from build123d import *

# Parameters (mm, degrees)
SKETCH_1_W          = 50
SKETCH_1_H          = 65
BOSS_EXTRUDE1_DEPTH = 20
SKETCH11_R          = 1.2
CUT_EXTRUDE1_DEPTH  = 28
SKETCH12_R          = 7
CUT_EXTRUDE2_DEPTH  = 15


with BuildPart() as part:
    # 草圖1 → Boss-Extrude1 (new body)
    with BuildSketch(Plane.XY):
        with Locations((2.083333333, 32.5)):
            Rectangle(SKETCH_1_W, SKETCH_1_H)
    extrude(amount=BOSS_EXTRUDE1_DEPTH)

    # Sketch11 → Cut-Extrude1 (cut)
    with BuildSketch(Plane.XY):
        with Locations((-2.916666667, 60.81)):
            Circle(SKETCH11_R)
        with Locations((-2.616666667, 13.19)):
            Circle(SKETCH11_R)
        with Locations((6.783333333, 13.19)):
            Circle(SKETCH11_R)
        with Locations((7.083333333, 60.81)):
            Circle(SKETCH11_R)
        Polygon((4.942250508, 65), (-0.775583841, 65), (-0.775583841, 58), (-8.416666667, 58), (-8.416666667, 16), (12.583333333, 16), (12.583333333, 58), (4.942250508, 58), align=None)
    extrude(amount=CUT_EXTRUDE1_DEPTH, mode=Mode.SUBTRACT)

    # Sketch12 → Cut-Extrude2 (cut)
    with BuildSketch(Plane(origin=(0, 0, 0), x_dir=(1, 0, 0), z_dir=(0, 1, 0))):
        with Locations((-15.232669486, -9.9188946)):
            Circle(SKETCH12_R)
        with Locations((18.767330514, -9.9188946)):
            Circle(SKETCH12_R)
    extrude(amount=CUT_EXTRUDE2_DEPTH, mode=Mode.SUBTRACT)


solid = part.part
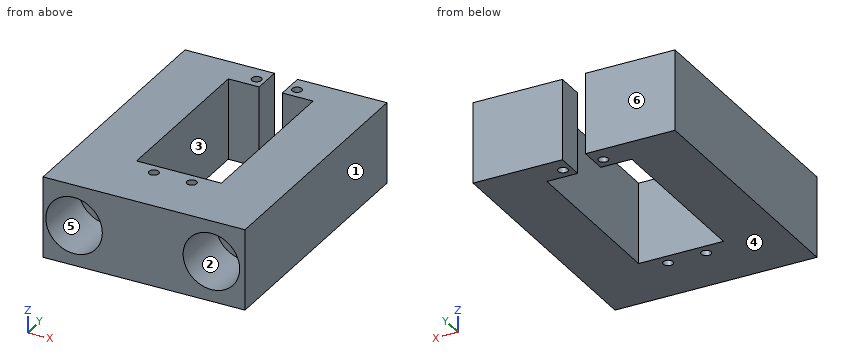
Work out the finished part from the listing and answer in its coordinate system (mm). Face numbers are marked on the shaded views. A direction names the side the tool comes from. Round coordinates to 2 decimals unless told otherwise and drop trailing zeros. Order: outer loops, then holes, each group sorted by start corner. A loop starts at its lowest first (then second) coordinate and runs counter-clockwise, first axis right, second up. Notation, with made-up numbers: M -23.75,63 L 1.25,63 A30 ccw 1.25,101 Z; hole C 22.5,43.5 d10. An arc over 180 degrees is marked long. One line per item, written item: value.
Q1. Determine the mould class of the marked faces 4, 5 and 6 for opening direction Z: released by +Z, released by -Z, zero draft, split by the parting line, or undercut.
Derived:
face 4: released by -Z
face 5: undercut
face 6: zero draft
Q2. Find section D-D on y = 13.19. Write down the section's boundary in (x, z), then the cut area to 3 significant figures.
Derived:
outline: M -22.92,0 L -3.82,0 L -3.82,20 L -22.92,20 Z; M -1.42,0 L 5.58,0 L 5.58,20 L -1.42,20 Z; M 7.98,0 L 27.08,0 L 27.08,20 L 7.98,20 Z; hole C -15.23,9.92 d14; hole C 18.77,9.92 d14
area: 596 mm²
Q3. Straight lines are drawn through the part: line 1 (X direction, y = 57.5, z = 2.25); line 2 (X direction, y = 11, z = 9.5); line 3 (Y direction, x = 6.5, z = 4). For each, find the intervals that lie inside material, in ascending order.
Derived:
line 1: -22.92 to -8.42, 12.58 to 27.08
line 2: -22.92 to -22.22, -8.25 to 11.78, 25.75 to 27.08
line 3: 0 to 12.02, 14.36 to 16, 58 to 59.76, 61.86 to 65
Q4. For the marked faces 1, 2 and 3, determine the directions among +Z, -Z, +X, -X, +Y, -Y from which every point of the face is accessible in a straight line to the end or side of a thin tool.
Derived:
face 1: +Z, -Z, +X, +Y, -Y
face 2: -Y
face 3: +Z, -Z
Q5. A flat-ended cylindrical pin translates along its axis: pin 1 (11 mm diameter, centred on x = 19, z = 9.5, fed in from -Y). Find the tip coordinate at first contact, or state that the pin passes through.
Derived:
pin 1: y = 15
Q6. Find section A-A on y = 23. Write down the section's boundary in (x, z).
Derived:
outline: M -22.92,0 L -8.42,0 L -8.42,20 L -22.92,20 Z; M 12.58,0 L 27.08,0 L 27.08,20 L 12.58,20 Z
Q7. Find section B-B on x = 10.5. Write down the section's boundary in (y, z).
Derived:
outline: M 0,0 L 16,0 L 16,20 L 0,20 Z; M 58,0 L 65,0 L 65,20 L 58,20 Z
Q8. Find section C-C on y = 60.81. Write down the section's boundary in (x, z), then the cut area to 3 significant figures.
Derived:
outline: M -22.92,0 L -4.12,0 L -4.12,20 L -22.92,20 Z; M -1.72,0 L -0.78,0 L -0.78,20 L -1.72,20 Z; M 4.94,0 L 5.88,0 L 5.88,20 L 4.94,20 Z; M 8.28,0 L 27.08,0 L 27.08,20 L 8.28,20 Z
area: 790 mm²
